Build history of the part. All positions in model axes, mm. Face numbers are marked on the shaded views. A direction names the side the tool comes from. Round coordinates to 2 decimals unless told otherwise and drop trailing zeros. Loops run counter-clockwise (first coordinate to the right, second up) from the corner with the lowest first, then second, coordinate; pieces in that order, holes last. Notation, with made-up numbers: (-20.5, -39.75) - (-3.5, -39.75) arc R24 cw to (-3.5, -0.75) - close; hole circle Ø6 at (68, -35.75). An arc over 180 degrees is marked (long way). Use a Markdown table: item, result.
from build123d import *

# Parameters (mm, degrees)
SKETCH1_W           = 20
SKETCH1_H           = 24
BOSS_EXTRUDE1_DEPTH = 3
SKETCH2_W           = 20
SKETCH2_H           = 24
SKETCH2_W_2         = 16
SKETCH2_H_2         = 21.5
BOSS_EXTRUDE2_DEPTH = 10
SKETCH3_W           = 9.25
SKETCH3_H           = 5.25
BOSS_EXTRUDE3_DEPTH = 2
CHAMFER1_SIZE       = 1
SKETCH4_W           = 6.75
SKETCH4_H           = 5.2
SKETCH4_R           = 1.5
BOSS_EXTRUDE4_DEPTH = 2
SKETCH5_W           = 16
SKETCH5_H           = 5.615862193
CUT_EXTRUDE1_DEPTH  = 33.887117539
SKETCH6_W           = 4.619985453
SKETCH6_H           = 12.899576223
CUT_EXTRUDE4_DEPTH  = 33.932696519


with BuildPart() as part:
    # Sketch1 → Boss-Extrude1 (new body)
    with BuildSketch(Plane.XY):
        Rectangle(SKETCH1_W, SKETCH1_H)
    extrude(amount=BOSS_EXTRUDE1_DEPTH)

    # Sketch2 → Boss-Extrude2 (add)
    with BuildSketch(Plane.XY.offset(3)):
        Rectangle(SKETCH2_W, SKETCH2_H)
        Rectangle(SKETCH2_W_2, SKETCH2_H_2, mode=Mode.SUBTRACT)
    extrude(amount=BOSS_EXTRUDE2_DEPTH)

    # Sketch3 → Boss-Extrude3 (add)
    with BuildSketch(Plane.XY.offset(13)):
        with Locations((0, 9.375)):
            Rectangle(SKETCH3_W, SKETCH3_H)
    extrude(amount=BOSS_EXTRUDE3_DEPTH)

    # Chamfer1
    chamfer1_edges = [part.edges().sort_by_distance(p)[0] for p in [
        (-4.625, 9.375, 15),
        (0, 6.75, 15),
        (4.625, 9.375, 15),
    ]]
    chamfer(chamfer1_edges, length=CHAMFER1_SIZE)

    # Sketch4 → Boss-Extrude4 (add)
    # profile 1 of 2: a face of its own
    with BuildSketch(Plane(origin=(0, 0, 0), x_dir=(-1, 0, 0), z_dir=(0, 0, -1))):
        with Locations((-13.375, 0)):
            Rectangle(SKETCH4_W, SKETCH4_H)
        with Locations((-14.25, 0)):
            Circle(SKETCH4_R, mode=Mode.SUBTRACT)
    # profile 2 of 2: a face of its own
    with BuildSketch(Plane(origin=(0, 0, 0), x_dir=(-1, 0, 0), z_dir=(0, 0, -1))):
        with Locations((13.375, 0)):
            Rectangle(SKETCH4_W, SKETCH4_H)
        with Locations((14.25, 0)):
            Circle(SKETCH4_R, mode=Mode.SUBTRACT)
    extrude(amount=-BOSS_EXTRUDE4_DEPTH)

    # Sketch5 → Cut-Extrude1 (cut, through all)
    with BuildSketch(Plane(origin=(0, 12, 0), x_dir=(1, 0, 0), z_dir=(0, 1, 0))):
        with Locations((0, -5.807931096)):
            Rectangle(SKETCH5_W, SKETCH5_H)
    extrude(amount=-CUT_EXTRUDE1_DEPTH, mode=Mode.SUBTRACT)

    # Sketch6 → Cut-Extrude4 (cut, through all)
    with BuildSketch(Plane.ZY.offset(10)):
        with Locations((5.309992727, 0.119967863)):
            Rectangle(SKETCH6_W, SKETCH6_H)
    extrude(amount=-CUT_EXTRUDE4_DEPTH, mode=Mode.SUBTRACT)


solid = part.part
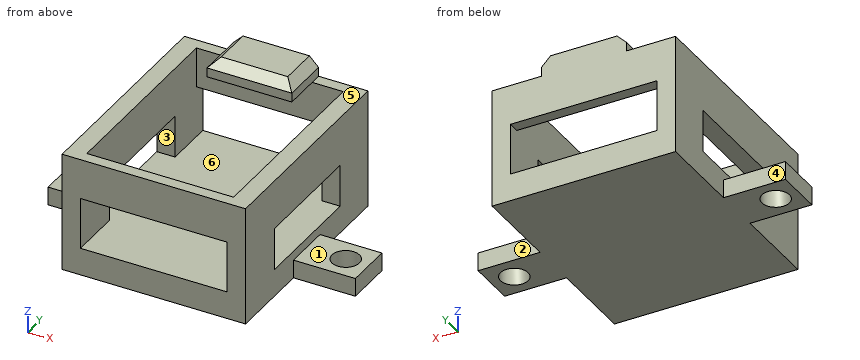
Q1. Pull direction Z, two halves, no side cores. Call the marked faces 4, 5 and 6: pulls with the +Z half, pulls with the -Z half, needs draft (parallel to the pull), parting line crosses it, or undercut.
Results found:
| item | result |
|---|---|
| face 4 | needs draft |
| face 5 | pulls with the +Z half |
| face 6 | undercut |
Q2. Probe line 1 (Y direction, x = -7, z = 12); line 2 (X direction, y = 4, z = 8); line 3 (Y direction, x = 14.25, z = 0.85). List the from-to ranges inside material, lowest first.
Results found:
| item | result |
|---|---|
| line 1 | y = -12 to -10.75, 10.75 to 12 |
| line 2 | x = -10 to -8, 8 to 10 |
| line 3 | y = -2.6 to -1.5, 1.5 to 2.6 |
Q3. Which spindle directions (+Z, -Z, +X, -X, +Y, -Y) get a long thin tool onto all of the face, cutting with end or side? Do the marked faces 1, 2 and 3. Say none if no direction does.
Results found:
| item | result |
|---|---|
| face 1 | +Z, +X, +Y, -Y |
| face 2 | +Z, -Z, +X, +Y |
| face 3 | +X, -X |
Q4. Cut at D-D, the plane x = 2. List the corners of the cut face in (y, z), plus the area to 3 significant figures.
Results found:
| item | result |
|---|---|
| outline | (-12, 0) - (12, 0) - (12, 3) - (-12, 3) - close; (-12, 8.62) - (-10.75, 8.62) - (-10.75, 13) - (-12, 13) - close; (6.75, 13) - (10.75, 13) - (10.75, 8.62) - (12, 8.62) - (12, 15) - (7.75, 15) - (6.75, 14) - close |
| area | 93.0 mm2 |
Q5. Cut at B-B, the plane x = 14.25. List the corners of the cut face in (y, z).
Results found:
| item | result |
|---|---|
| outline | (-2.6, 0) - (-1.5, 0) - (-1.5, 2) - (-2.6, 2) - close; (1.5, 0) - (2.6, 0) - (2.6, 2) - (1.5, 2) - close |
Q6. Cut at C-C, the plane z = 9.5. List the corners of the cut face in (x, y), plus the area to 3 significant figures.
Results found:
| item | result |
|---|---|
| outline | (-10, -12) - (10, -12) - (10, 12) - (-10, 12) - close; hole (-8, -10.75) - (8, -10.75) - (8, 10.75) - (-8, 10.75) - close |
| area | 136 mm2 |
Q7. Drop flat-ended pins along their axis: pin 1 (6 mm diameter, centred on y = 2.5, z = 7.5, fed in from -X); pin 2 (6 mm diameter, centred on y = -6, z = 11, fed in from +X); pin 3 (0.8 mm diameter, centred on y = 10.5, z = 13.5, fed in from -X) (3 decimals). Give the stop position or say it passes through.
Results found:
| item | result |
|---|---|
| pin 1 | stops at x = -10 |
| pin 2 | stops at x = 10 |
| pin 3 | stops at x = -4.625 |
Q8. Cut at A-A, the plane y = -4.5. List the corners of the cut face in (x, z), plus the area to 3 significant figures.
Results found:
| item | result |
|---|---|
| outline | (-10, 0) - (10, 0) - (10, 3) - (-10, 3) - close; (-10, 7.62) - (-8, 7.62) - (-8, 13) - (-10, 13) - close; (8, 7.62) - (10, 7.62) - (10, 13) - (8, 13) - close |
| area | 81.5 mm2 |
